```python
from build123d import *

# Parameters (mm, degrees)
SKETCH1_W           = 342.9
SKETCH1_H           = 139.7
BOSS_EXTRUDE1_DEPTH = 12.7
SKETCH3_R           = 1.5
SKETCH3_R_2         = 1.500000048
CUT_EXTRUDE1_DEPTH  = 13.7
SKETCH4_W           = 17.78
SKETCH4_H           = 101.6
SKETCH4_W_2         = 101.6
SKETCH4_H_2         = 17.78
CUT_EXTRUDE2_DEPTH  = 13.7
SKETCH5_R           = 1.5
CUT_EXTRUDE3_DEPTH  = 13.7


with BuildPart() as part:
    # Sketch1 → Boss-Extrude1 (new body)
    with BuildSketch(Plane(origin=(0, 0, 0), x_dir=(1, 0, 0), z_dir=(0, 1, 0))):
        with Locations((171.45, 69.85)):
            Rectangle(SKETCH1_W, SKETCH1_H)
    extrude(amount=BOSS_EXTRUDE1_DEPTH)

    # Sketch3 → Cut-Extrude1 (cut, through all)
    with BuildSketch(Plane(origin=(0, 12.7, 0), x_dir=(1, 0, 0), z_dir=(0, 1, 0))):
        with Locations((330.2, 82.55)):
            Circle(SKETCH3_R)
        with Locations((330.2, 57.15)):
            Circle(SKETCH3_R_2)
        with Locations((304.8, 57.15)):
            Circle(SKETCH3_R)
        with Locations((304.8, 82.55)):
            Circle(SKETCH3_R_2)
    cut_extrude1 = extrude(amount=-CUT_EXTRUDE1_DEPTH, mode=Mode.SUBTRACT)

    # Mirror1: Cut-Extrude1 across plane
    add(cut_extrude1.mirror(Plane.ZY.offset(-171.45)), mode=Mode.SUBTRACT)

    # Sketch4 → Cut-Extrude2 (cut, through all)
    with BuildSketch(Plane(origin=(0, 12.7, 0), x_dir=(1, 0, 0), z_dir=(0, 1, 0))):
        with Locations((270.51, 69.85)):
            Rectangle(SKETCH4_W, SKETCH4_H)
        with Locations((142.875, 69.85)):
            Rectangle(SKETCH4_W_2, SKETCH4_H_2)
    extrude(amount=-CUT_EXTRUDE2_DEPTH, mode=Mode.SUBTRACT)

    # Sketch5 → Cut-Extrude3 (cut, through all)
    with BuildSketch(Plane(origin=(0, 12.7, 0), x_dir=(1, 0, 0), z_dir=(0, 1, 0))):
        with Locations((130.175, 127)):
            Circle(SKETCH5_R)
        with Locations((155.575, 127)):
            Circle(SKETCH5_R)
        with Locations((155.575, 101.6)):
            Circle(SKETCH5_R)
        with Locations((130.175, 101.6)):
            Circle(SKETCH5_R)
    cut_extrude3 = extrude(amount=-CUT_EXTRUDE3_DEPTH, mode=Mode.SUBTRACT)

    # Mirror3: Cut-Extrude3 across plane
    add(cut_extrude3.mirror(Plane(origin=(0, 0, -69.85), x_dir=(1, 0, 0), z_dir=(0, 0, -1))), mode=Mode.SUBTRACT)


solid = part.part
```
The listing builds one solid part. Answer for the finished solid, in the listing's coordinates (mm). A direction names the side the tool comes from. Round coordinates to 2 decimals unless told otherwise and drop trailing zeros. Loops run counter-clockwise (first coordinate to the right, second up) from the corner with the lowest first, then second, coordinate; pieces in that order, holes last.
Q1. Section D-D, the plane x = 124.5 is taken. Determine the outline of the cut face in (y, z), then the cut area to 3 significant figures.
Q2. For a pull along Z with two mould halves and no side action, classify faces 1 (the face through (169, 6, 0)), 2 (the face through (169, 0, -55)), 3 (the face through (142, 6, -78.74)) as released by +Z, released by -Z, zero draft, split by the parting line, or undercut.
Q3. Section A-A, the plane x = 272 is taken. Determine the outline of the cut face in (y, z), then the cut area to 3 significant figures.
Q4. Section B-B, the plane z = -75.5 is taken. Determine the outline of the cut face in (x, y) (3 decimals).
Q5. Section C-C, the plane y = 5.5 is taken. Count the separate pieces of the cut face and the enclosed holes in it, then the cut area to 3 significant figures.
Q6. Which of the six approach directions +Z, -Z, +X, -X, +Y, -Y give full straight-line access (tool end or side, diameter ignored) to faces 4 (the face through (0, 6, -69)), 5 (the face through (92.075, 6, -70))?
Q7. Find the intervals of material crossed by line 1 (X direction, y = 3.5, z = -57.15); line 2 (X direction, y = 4, z = -101.6) (3 decimals); line 3 (Z direction, x = 304.8, y = 7.75), in increasing order.
Completed:
1. outline: (0, -139.7) - (12.7, -139.7) - (12.7, -78.74) - (0, -78.74) - close; (0, -60.96) - (12.7, -60.96) - (12.7, 0) - (0, 0) - close
1. area: 1,550 mm2
2. face 1: released by +Z
2. face 2: zero draft
2. face 3: undercut
3. outline: (0, -139.7) - (12.7, -139.7) - (12.7, -120.65) - (0, -120.65) - close; (0, -19.05) - (12.7, -19.05) - (12.7, 0) - (0, 0) - close
3. area: 484 mm2
4. outline: (0, 0) - (92.075, 0) - (92.075, 12.7) - (0, 12.7) - close; (193.675, 0) - (261.62, 0) - (261.62, 12.7) - (193.675, 12.7) - close; (279.4, 0) - (342.9, 0) - (342.9, 12.7) - (279.4, 12.7) - close
5. separate pieces: 1
5. enclosed holes: 18
5. area: 44,200 mm2
6. face 4: +Z, -Z, -X, +Y, -Y
6. face 5: +Y, -Y
7. line 1: x = 0 to 11.2, 14.2 to 36.6, 39.6 to 261.62, 279.4 to 303.3, 306.3 to 328.7, 331.7 to 342.9
7. line 2: x = 0 to 128.675, 131.675 to 154.075, 157.075 to 261.62, 279.4 to 342.9
7. line 3: z = -139.7 to -84.05, -81.05 to -58.65, -55.65 to 0
